from build123d import *

# Parameters (mm, degrees)
SKETCH3_W               = 6
SKETCH3_H               = 2
BOSS_EXTRUDE4_DEPTH     = 1
SKETCH4_W               = 6
SKETCH4_H               = 2
BOSS_EXTRUDE5_DEPTH     = 1
CUT_EXTRUDE2_DEPTH      = 4
CUT_EXTRUDE2_DEPTH_BACK = 4
SKETCH6_R               = 1.5
CUT_EXTRUDE3_DEPTH      = 18
SKETCH7_OUTSIDE_W       = 11.98
SKETCH7_OUTSIDE_H       = 11.98
SKETCH7_OUTSIDE_R       = 3
CUT_EXTRUDE4_DEPTH      = 10.0000001
CUT_EXTRUDE4_DEPTH_BACK = 10.0000001


with BuildPart() as part:
    # Sketch1 → Revolve5 (revolve)
    with BuildSketch(Plane.XY):
        Polygon((0, 9), (-2.5, 9), (-2.5, 8.5), (-2, 8.5), (-2, 0.5), (-2.25, 0.5), (-2.25, -0.5), (-2, -0.5), (-2, -8.5), (-2.5, -8.5), (-2.5, -9), (0, -9), align=None)
    revolve(axis=Axis((0, 9, 0), (0, -1, 0)))

    # Sketch3 → Boss-Extrude4 (add, symmetric)
    with BuildSketch(Plane.XY):
        with Locations((0, 1)):
            Rectangle(SKETCH3_W, SKETCH3_H)
    extrude(amount=BOSS_EXTRUDE4_DEPTH, both=True)

    # Sketch4 → Boss-Extrude5 (add, symmetric)
    with BuildSketch(Plane(origin=(0, 0, 0), x_dir=(0, 0, -1), z_dir=(1, 0, 0))):
        with Locations((0, -1)):
            Rectangle(SKETCH4_W, SKETCH4_H)
    extrude(amount=BOSS_EXTRUDE5_DEPTH, both=True)

    # Sketch5 → Cut-Extrude2 (cut, two sides)
    with BuildSketch(Plane.XY) as cut_extrude2_sk:
        with BuildLine():
            Line((-1, 9), (-1, 6))
            ThreePointArc((-1, 6), (0, 5), (1, 6))
            Line((1, 6), (1, 9))
            Line((1, 9), (-1, 9))
        make_face()
        with BuildLine():
            Line((-1, -9), (-1, -6))
            ThreePointArc((-1, -6), (0, -5), (1, -6))
            Line((1, -6), (1, -9))
            Line((1, -9), (-1, -9))
        make_face()
    extrude(amount=CUT_EXTRUDE2_DEPTH, mode=Mode.SUBTRACT)
    extrude(cut_extrude2_sk.sketch, amount=-CUT_EXTRUDE2_DEPTH_BACK, mode=Mode.SUBTRACT)

    # Sketch6 → Cut-Extrude3 (cut)
    with BuildSketch(Plane(origin=(0, 9, 0), x_dir=(1, 0, 0), z_dir=(0, 1, 0))):
        Circle(SKETCH6_R)
    extrude(amount=-CUT_EXTRUDE3_DEPTH, mode=Mode.SUBTRACT)

    # Sketch7 outside → Cut-Extrude4 (cut, two sides)
    with BuildSketch(Plane(origin=(0, 0, 0), x_dir=(1, 0, 0), z_dir=(0, 1, 0))) as cut_extrude4_sk:
        Rectangle(SKETCH7_OUTSIDE_W, SKETCH7_OUTSIDE_H)
        Circle(SKETCH7_OUTSIDE_R, mode=Mode.SUBTRACT)
    extrude(amount=CUT_EXTRUDE4_DEPTH, mode=Mode.SUBTRACT)
    extrude(cut_extrude4_sk.sketch, amount=-CUT_EXTRUDE4_DEPTH_BACK, mode=Mode.SUBTRACT)


solid = part.part
Can you work these out from the model? Positions are in its coordinate system, mm. A direction names the side the tool comes from. Give positions to 0.01 mm unless a question says otherwise; leave off trailing zeros. Loops run counter-clockwise (first coordinate to the right, second up) from the corner with the lowest first, then second, coordinate; pieces in that order, holes last. Notation, with made-up numbers: (59, -38) - (112, -38) arc R32 cw to (112, 0) - close; hole circle Ø9 at (57, 77.25). An arc over 180 degrees is marked (long way). Answer as a JSON object with one key per item and string values.
Q1. Imagine slicing it at B-B on x = 0. Write out the boundary of the cut face in (y, z).
Geometry says:
{"outline": "(-5, -2) - (-2, -2) - (-2, -3) - (0, -3) - (0, -2.25) - (0.5, -2.25) - (0.5, -2) - (5, -2) - (5, -1.5) - (-5, -1.5) - close; (-5, 1.5) - (5, 1.5) - (5, 2) - (0.5, 2) - (0.5, 2.25) - (0, 2.25) - (0, 3) - (-2, 3) - (-2, 2) - (-5, 2) - close"}
Q2. If I drill on L1, parallel to Y at x = 2.3, z = 0.8; L2, parallel to Z at x = 0, y = -1.5; L3, parallel to X at y = 4.5, z = 0, over which ranges is the centre line in solid material (lowest first)?
Geometry says:
{"L1": "-9 to -8.5, 0 to 2, 8.5 to 9", "L2": "-3 to -1.5, 1.5 to 3", "L3": "-2 to -1.5, 1.5 to 2"}
Q3. Imagine slicing it at D-D on z = -0.7. Write out the boundary of the cut face in (x, y), plus the area to 3 significant figures.
Geometry says:
{"outline": "(-2.92, 0) - (-2.14, 0) - (-2.14, -0.5) - (-1.87, -0.5) - (-1.87, -8.5) - (-2.4, -8.5) - (-2.4, -9) - (-1.33, -9) - (-1.33, 9) - (-2.4, 9) - (-2.4, 8.5) - (-1.87, 8.5) - (-1.87, 2) - (-2.92, 2) - close; (1.33, -9) - (2.4, -9) - (2.4, -8.5) - (1.87, -8.5) - (1.87, -0.5) - (2.14, -0.5) - (2.14, 0) - (2.92, 0) - (2.92, 2) - (1.87, 2) - (1.87, 8.5) - (2.4, 8.5) - (2.4, 9) - (1.33, 9) - close", "area": "25.2 mm²"}
Q4. Will these pins go through, and if not, where does the flat tip stop? P1, Ø1, axis at y = -4, z = 0.5, coming from the +X side; P2, Ø1.8, axis at x = 0, z = 0, coming from the -Y side; P3, Ø1, axis at x = -1, y = -1.5, coming from the +Z side; P4, Ø1.5, axis at y = -5, z = 1.5, coming from the -X side.
Geometry says:
{"P1": "x = 2", "P2": "through", "P3": "z = 2.96", "P4": "x = -1.85"}
Q5. Imagine slicing it at A-A on z = 0. Write out the boundary of the cut face in (x, y), plus the area to 4 significant figures.
Geometry says:
{"outline": "(-3, 0) - (-2.25, 0) - (-2.25, -0.5) - (-2, -0.5) - (-2, -8.5) - (-2.5, -8.5) - (-2.5, -9) - (-1.5, -9) - (-1.5, 9) - (-2.5, 9) - (-2.5, 8.5) - (-2, 8.5) - (-2, 2) - (-3, 2) - close; (1.5, -9) - (2.5, -9) - (2.5, -8.5) - (2, -8.5) - (2, -0.5) - (2.25, -0.5) - (2.25, 0) - (3, 0) - (3, 2) - (2, 2) - (2, 8.5) - (2.5, 8.5) - (2.5, 9) - (1.5, 9) - close", "area": "23.25 mm²"}
Q6. If we mould it in two halves opening along Y, with no side actions, what happens to faces 6 (the flat face through (1, 7.5, 1.4)), 7 (the flat face through (1, -1, -2)), 8 (the cylindrical face through (2.248, -0.229, -0.099)), 9 (the flat face through (2, 9, 0))? For each: pulls with the +Y half, pulls with the -Y half, needs draft (parallel to the pull), parting line crosses it, or undercut.
Geometry says:
{"face 6": "needs draft", "face 7": "undercut", "face 8": "undercut", "face 9": "pulls with the +Y half"}
Q7. Imagine slicing it at C-C on y = 3.25. Write out the boundary of the cut face in (x, z), plus the area to 3 significant figures.
Geometry says:
{"outline": "circle Ø4 at (0, 0); hole circle Ø3 at (0, 0)", "area": "5.50 mm²"}
Q8. Which directions (+Z, -Z, +X, -X, +Y, -Y) give clear straight access to the entire face, cutting with the end or side of a thin tool? Please do faces 1 (the flat face through (1, -1, 2)), 2 (the cylindrical face through (1.474, 4.444, -1.352)), 3 (the flat face through (1, -7.5, 1.5)), 4 (the flat face through (-2.2, 8.5, 0.2)), 5 (the cylindrical face through (-2.5, -8.8, 0)).
Geometry says:
{"face 1": "+Z, +X", "face 2": "none", "face 3": "+Z, -Z, -Y", "face 4": "-X", "face 5": "-X, -Y"}
